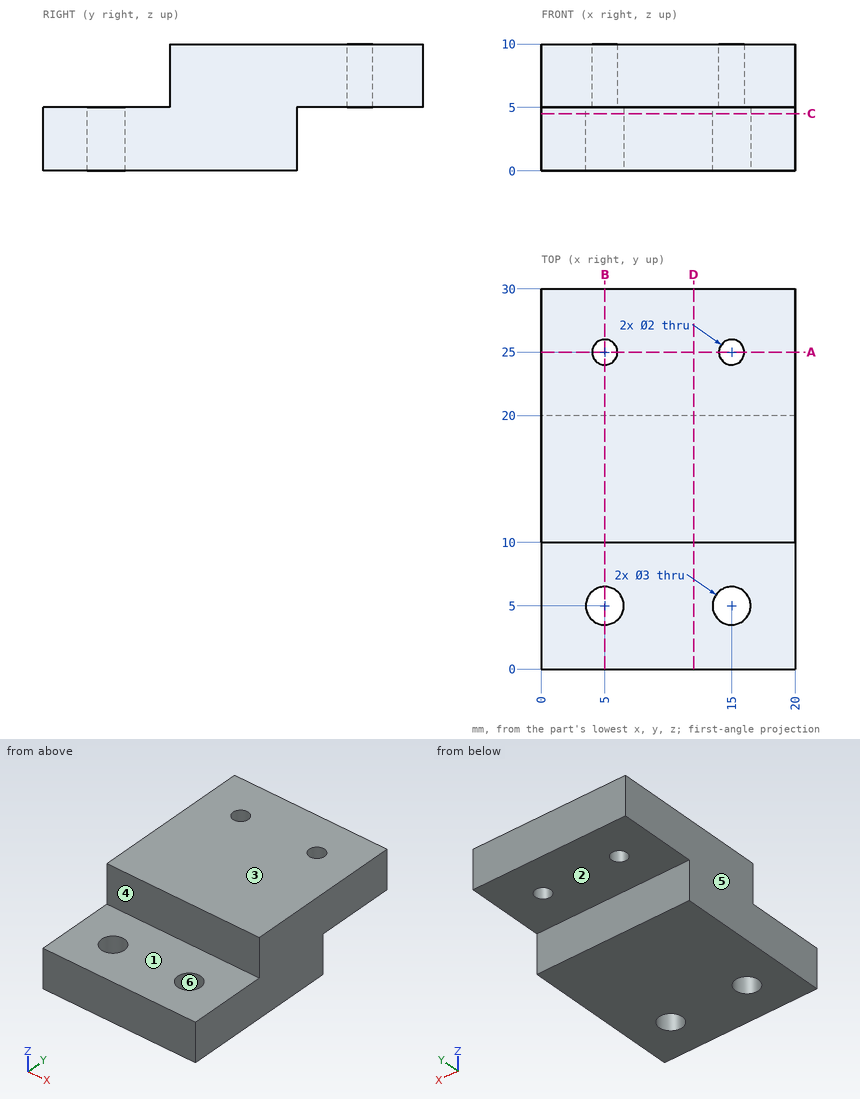
The figure shows three views and two pictorial views of one solid part (mm, origin at its lowest corner). Answer the questions. A direction names the side the tool comes from. Coordinates: 2 decimals unless noted, no trailing zeros. Loops run counter-clockwise (first coordinate to the right, second up) from the corner with the lowest first, then second, coordinate; pieces in that order, holes last. Notation, with made-up numbers: (-13, 17) -> (2, 17) arc R17 cw to (2, 41) -> close; hole circle Ø1 at (71, 69). An arc over 180 degrees is marked (long way). Return JSON: item names as keys, results as strings. Group by question number.
(1) Given pin 1 Ø1.5 at (x, z) = (14, 6.5) entering from -Y; pin 2 Ø8 at (x, y) = (6, 4.5) entering from +Z; pin 3 Ø8 at (x, y) = (10, 25.5) entering from -Z, each flat-ended and moving along its own axis, determine where each tip first touches the part or whether it passes through.
(2) A cutting plane is placed at A-A on y = 25. Write down the section's boundary in (x, z).
(3) A cutting plane is placed at D-D on x = 12. Write down the section's boundary in (y, z).
(4) A cutting plane is placed at B-B on x = 5. Write down the section's boundary in (y, z).
(5) Which of the six approach directions +Z, -Z, +X, -X, +Y, -Y give full straight-line access (tool end or side, diameter ignored) to the marked faces 1, 2 and 3?
(6) Determine the mould class of the marked faces 4, 5 and 6 for opening direction X: released by +X, released by -X, zero draft, split by the parting line, or undercut.
(7) Find the intervals of material crossed by probe 1 along Y at (x, z) = (15, 7.7); probe 2 along Y at (x, z) = (15, 3.6); probe 3 along Z at (x, y) = (5.5, 20.5), in increasing order. Write a range as from..to.
(8) A cutting plane is placed at C-C on z = 4.5. Write down the section's boundary in (x, y), and give its area (3 significant figures).
The answers:
{
 "1": {"pin 1": "stops at y = 10", "pin 2": "stops at z = 5", "pin 3": "stops at z = 5"},
 "2": {"outline": "(0, 5) -> (4, 5) -> (4, 10) -> (0, 10) -> close; (6, 5) -> (14, 5) -> (14, 10) -> (6, 10) -> close; (16, 5) -> (20, 5) -> (20, 10) -> (16, 10) -> close"},
 "3": {"outline": "(0, 0) -> (20, 0) -> (20, 5) -> (30, 5) -> (30, 10) -> (10, 10) -> (10, 5) -> (0, 5) -> close"},
 "4": {"outline": "(0, 0) -> (3.5, 0) -> (3.5, 5) -> (0, 5) -> close; (6.5, 0) -> (20, 0) -> (20, 5) -> (24, 5) -> (24, 10) -> (10, 10) -> (10, 5) -> (6.5, 5) -> close; (26, 5) -> (30, 5) -> (30, 10) -> (26, 10) -> close"},
 "5": {"face 1": "+Z, +X, -X, -Y", "face 2": "-Z, +X, -X, +Y", "face 3": "+Z, +X, -X, +Y, -Y"},
 "6": {"face 4": "zero draft", "face 5": "released by -X", "face 6": "undercut"},
 "7": {"probe 1": "y = 10..24, 26..30", "probe 2": "y = 0..3.5, 6.5..20", "probe 3": "z = 5..10"},
 "8": {"outline": "(0, 0) -> (20, 0) -> (20, 20) -> (0, 20) -> close; hole circle Ø3 at (5, 5); hole circle Ø3 at (15, 5)", "area": "386 mm^2"}
}
